Check sheet for the modelled part. Datum: model origin and axes. Units: mm. Face numbers are marked on the shaded views. Round coordinates to 2 decimals unless told otherwise and drop trailing zeros. Loops run counter-clockwise (first coordinate to the right, second up) from the corner with the lowest first, then second, coordinate; pieces in that order, holes last. Notation, with made-up numbers: (-35.75, 20.5) - (-13.75, 20.5) arc R23 ccw to (-13.75, 52.5) - close; hole circle Ø5 at (14, -34.5). An arc over 180 degrees is marked (long way). Put each result on its own line as item: value. Start each with the question number.
Item 1: Material ranges on line 1 along Z through (x, y) = (-0.25, 1.05); line 2 along X through (y, z) = (1.9, -4); line 3 along X through (y, z) = (2.55, 3.25), recorded low to high.
Item 2: Section check A-A, the plane x = -1.5. Record the cut outline in (y, z).
Item 3: Section check B-B, the plane y = 0.55. Record the cut outline in (x, z) (3 decimals).
Item 4: Gauge pin test, flat end, axial feed: pin 1 Ø2 at (x, z) = (-6, 3.5) entering from -Y. Record the tip position at first contact, or that the pin passes through.
Item 5: Draft check along Z on the marked faces 1, 2, 3 and 4. Enter one of: pulls with the +Z half, pulls with the -Z half, needs draft (parallel to the pull), parting line crosses it, or undercut.
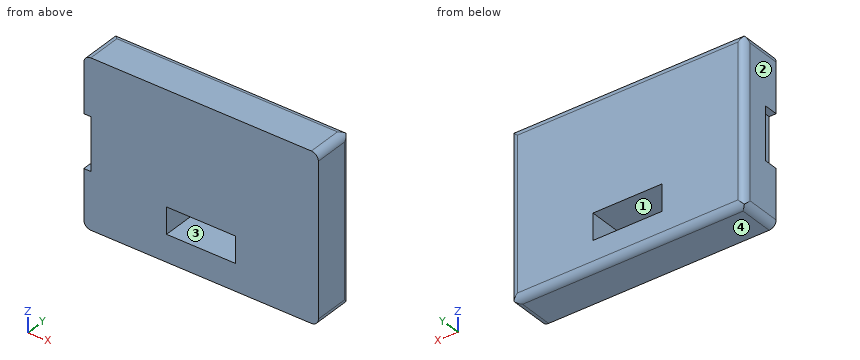
Autodesk Inventor part; units mm, degrees
ref_plane "P_XY" through (0, 0, 0) normal (0, 1, 0) x (1, 0, 0)
ref_plane "P_YZ" through (0, 0, 0) normal (1, 0, 0) x (0, 0, -1)
ref_plane "P_ZX" through (0, 0, 0) normal (0, 0, -1) x (0, 1, 0)
sketch "Sketch_1" plane through (0, 0, 0) normal (0, 1, 0) x (-1, 0, 0)
  line L0 (8.4963, -5.4864) -> (8.4963, 5.4864)
  arc A0 (8.4963, 5.4864) -> (7.9883, 5.9944) centre (7.9883, 5.4864) ccw
  line L1 (7.9883, 5.9944) -> (-7.9883, 5.9944)
  arc A1 (-7.9883, 5.9944) -> (-8.4963, 5.4864) centre (-7.9883, 5.4864) ccw
  line L2 (-8.4963, 5.4864) -> (-8.4963, -5.4864)
  arc A2 (-8.4963, -5.4864) -> (-7.9883, -5.9944) centre (-7.9883, -5.4864) ccw
  line L3 (-7.9883, -5.9944) -> (7.9883, -5.9944)
  arc A3 (7.9883, -5.9944) -> (8.4963, -5.4864) centre (7.9883, -5.4864) ccw
extrude "Extrusion1" add sketch "Sketch_1" along normal blind 2.9972
sketch "Sketch_6" plane through (0, 0, 0) normal (0, 0, 1) x (1, 0, 0)
  line L0 (-10.16, 5.08) -> (-10.16, -2.54)
  line L1 (-10.16, -2.54) -> (10.16, -2.54)
  line L2 (10.16, -2.54) -> (10.16, 5.08)
  line L3 (10.16, 5.08) -> (-10.16, 5.08)
  line L4 (-8.4963, 0) -> (8.4963, 0)
  line L5 (8.4963, 0) -> (8.4963, 2.4892)
  arc A0 (8.4963, 2.4892) -> (7.9883, 2.9972) centre (7.9883, 2.4892) ccw
  line L6 (7.9883, 2.9972) -> (-7.9883, 2.9972)
  arc A1 (-7.9883, 2.9972) -> (-8.4963, 2.4892) centre (-7.9883, 2.4892) ccw
  line L7 (-8.4963, 2.4892) -> (-8.4963, 0)
extrude "Extrusion2" cut sketch "Sketch_6" along normal mid plane 15.24
sketch "Sketch_9" plane through (0, 0, 0) normal (1, 0, 0) x (0, 1, 0)
  line L0 (5.08, 10.16) -> (-2.54, 10.16)
  line L1 (-2.54, 10.16) -> (-2.54, -10.16)
  line L2 (-2.54, -10.16) -> (5.08, -10.16)
  line L3 (5.08, -10.16) -> (5.08, 10.16)
  line L4 (0, 5.9944) -> (0, -5.9944)
  line L5 (0, -5.9944) -> (2.4892, -5.9944)
  arc A0 (2.4892, -5.9944) -> (2.9972, -5.4864) centre (2.4892, -5.4864) ccw
  line L6 (2.9972, -5.4864) -> (2.9972, 5.4864)
  arc A1 (2.9972, 5.4864) -> (2.4892, 5.9944) centre (2.4892, 5.4864) ccw
  line L7 (2.4892, 5.9944) -> (0, 5.9944)
extrude "Extrusion3" cut sketch "Sketch_9" along normal mid plane 20.32
sketch "Sketch_4" plane through (-8.4963, 0, 0) normal (1, 0, 0) x (0, 0, -1)
  line L0 (-1.905, 0) -> (1.905, 0)
  line L1 (1.905, 0) -> (1.905, 1.016)
  line L2 (1.905, 1.016) -> (-1.905, 1.016)
  line L3 (-1.905, 1.016) -> (-1.905, 0)
extrude "Extrusion4" cut sketch "Sketch_4" along normal blind 0.508
sketch "Sketch_5" plane through (0, 0, 0) normal (0, 1, 0) x (-1, 0, 0)
  line L0 (2.5019, -4.0513) -> (2.5019, -2.1463)
  line L1 (2.5019, -2.1463) -> (-2.5019, -2.1463)
  line L2 (-2.5019, -2.1463) -> (-2.5019, -4.0513)
  line L3 (-2.5019, -4.0513) -> (2.5019, -4.0513)
extrude "Extrusion5" cut sketch "Sketch_5" along normal blind 5.08
ref_plane "P_XY" through (0, 0, 0) normal (0, 1, 0) x (1, 0, 0)
ref_plane "P_YZ" through (0, 0, 0) normal (1, 0, 0) x (0, 0, -1)
ref_plane "P_ZX" through (0, 0, 0) normal (0, 0, -1) x (0, 1, 0)
ref_plane "SPOT_XY" through (0, 0, -3.0988) normal (0, -1, 0) x (1, 0, 0)
ref_plane "SPOT_YZ" through (0, 0, -3.0988) normal (1, 0, 0) x (0, 0, 1)
ref_plane "SPOT_ZX" through (0, 0, -3.0988) normal (0, 0, 1) x (0, -1, 0)
properties part number "UB16NKG015F-NR"
Check result:
1. line 1: -5.99 to -4.05, -2.15 to 5.99
1. line 2: -8.5 to -2.5, 2.5 to 8.5
1. line 3: -8.49 to 8.49
2. outline: (0, -5.99) - (2.49, -5.99) arc R0.51 ccw to (3, -5.49) - (3, -4.05) - (0, -4.05) - close; (0, -2.15) - (3, -2.15) - (3, 5.49) arc R0.51 ccw to (2.49, 5.99) - (0, 5.99) - close
3. outline: (-8.496, -5.486) arc R0.508 ccw to (-7.988, -5.994) - (7.988, -5.994) arc R0.508 ccw to (8.496, -5.486) - (8.496, 5.486) arc R0.508 ccw to (7.988, 5.994) - (-7.988, 5.994) arc R0.508 ccw to (-8.496, 5.486) - (-8.496, 1.905) - (-7.988, 1.905) - (-7.988, -1.905) - (-8.496, -1.905) - close; hole (-2.502, -4.051) - (2.502, -4.051) - (2.502, -2.146) - (-2.502, -2.146) - close
4. pin 1: y = 0
5. face 1: undercut
5. face 2: needs draft
5. face 3: undercut
5. face 4: pulls with the -Z half
